Geometry check sheet. Reference: the model listing, model coordinates, mm. Face numbers are marked on the shaded views. A direction names the side the tool comes from. Give positions to 0.01 mm unless a question says otherwise; leave off trailing zeros. Loops run counter-clockwise (first coordinate to the right, second up) from the corner with the lowest first, then second, coordinate; pieces in that order, holes last. Notation, with made-up numbers: (81.25, -33.5) -> (116.25, -33.5) arc R27 cw to (116.25, -3.5) -> close; hole circle Ø11 at (44, -3). An arc over 180 degrees is marked (long way). One line per question, with ' | ' between items.
from build123d import *

# Parameters (mm, degrees)
F0_R     = 11
F1_DEPTH = 2
F2_R     = 4.5
F3_DEPTH = 0.5
F4_R     = 3.995
F5_DEPTH = 2.5


# Not quite as in the source:
# - a fillet or chamfer that OpenCascade refuses, or shapes differently, is made with other operations: its cross-section is extruded or revolved along the edge and cut away or added


with BuildPart() as f1:
    # F0 (on Top) → F1 (new body)
    with BuildSketch(Plane.XY):
        with Locations((-124.7583553195, 13.61318212)):
            Circle(F0_R)
    extrude(amount=F1_DEPTH)

    # F2 (on face) → F3 (join)
    with BuildSketch(Plane.XY.offset(2)):
        with Locations((-124.7583553195, 13.61318212)):
            Circle(F2_R)
    extrude(amount=F3_DEPTH)

    # F4 (on face) → F5 (join)
    with BuildSketch(Plane.XY.offset(2.5)):
        with Locations((-124.7583553195, 13.61318212)):
            Circle(F4_R)
    extrude(amount=F5_DEPTH)

    # F6: fillet of radius 2 on 2 edges, made by hand

    # F6_s1 → F6_t2 (revolve)
    with BuildSketch(Plane.XZ.offset(-13.61318212)):
        with BuildLine():
            ThreePointArc((-118.9351147195, 1.9996), (-119.642533578, 2.1287949759), (-120.2586198399, 2.4996999517))
            Line((-120.2586198399, 2.4996999517), (-120.3909703519, 2.3495733784))
            ThreePointArc((-120.3909703519, 2.3495733784), (-120.458491888, 2.2498499759), (-120.458491888, 2))
            Line((-120.458491888, 2), (-120.2583553195, 1.7998634315))
            ThreePointArc((-120.2583553195, 1.7998634315), (-119.5967350195, 1.7998634315), (-118.9351147195, 1.7994634315))
            Line((-118.9351147195, 1.7994634315), (-118.9351147195, 1.9996))
        make_face()
    revolve(axis=Axis((-124.7583553195, 13.61318212, 2), (0, 0, 1)))

    # F6_s3 → F6_t4 (revolve, cut)
    with BuildSketch(Plane.XZ.offset(-13.61318212)):
        with BuildLine():
            ThreePointArc((-113.7579553195, 1.999999807), (-114.3444830549, 0.5854449892), (-115.7593207719, -0.0004))
            Line((-115.7593207719, -0.0004), (-115.7593207719, -0.2005365685))
            ThreePointArc((-115.7593207719, -0.2005365685), (-114.7588380457, -0.2001365685), (-113.7583553195, -0.2001365685))
            Line((-113.7583553195, -0.2001365685), (-113.558218751, 0))
            ThreePointArc((-113.558218751, 0), (-113.558218751, 0.9999999035), (-113.5578187743, 1.9999032191))
            Line((-113.5578187743, 1.9999032191), (-113.7579553195, 1.999999807))
        make_face()
    revolve(axis=Axis((-124.7583553195, 13.61318212, 0), (0, 0, 1)), mode=Mode.SUBTRACT)


solid = f1.part
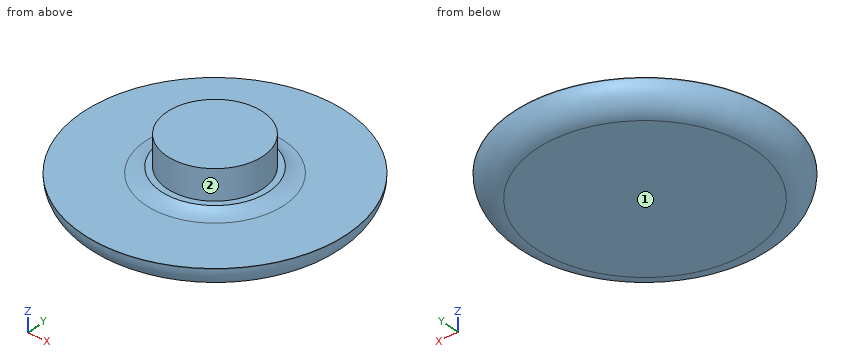
Item 1: Depth check by flat-ended pin: pin 1 Ø3 at (x, z) = (-129.5, 0.5) entering from +Y; pin 2 Ø5 at (x, y) = (-126.5, 11) entering from -Z; pin 3 Ø1.5 at (x, z) = (-128, 4) entering from -Y; pin 4 Ø1 at (x, z) = (-129.5, 2) entering from +Y. Enter the tip coordinate at first touch or a pass-through.
Result:
pin 1: y = 23.93 | pin 2: z = 0 | pin 3: y = 10.49 | pin 4: y = 23.76
Item 2: Sectioned sample at A-A (z = 0.55). Record the cut outline in (x, y) (1 decimal), plus the area to 3 significant figures.
Result:
outline: circle Ø20.8 at (-124.8, 13.6) | area: 338 mm2
Item 3: Scan lines: probe 1 along Z at (x, y) = (-121.5, 7.75); probe 2 along X at (y, z) = (13.75, 3.7); probe 3 along X at (y, z) = (13.5, 1.85). Record each from-to range of solid material in increasing order.
Result:
probe 1: 0 to 2 | probe 2: -128.75 to -120.77 | probe 3: -135.75 to -113.76
Item 4: Set-up check for the marked faces 1 and 2: record each of +Z, -Z, +X, -X, +Y, -Y from which the full face is reachable in a straight line by a thin tool's end or side.
Result:
face 1: -Z, +X, -X, +Y, -Y | face 2: +Z
Item 5: Sectioned sample at B-B (z = 3.5). Record the cut outline in (x, y) (3 decimals), plus the area to 3 significant figures.
Result:
outline: circle Ø7.99 at (-124.758, 13.613) | area: 50.1 mm2
